For this review, take the finished solid that the model builds, in its own axes (mm). Face numbers are marked on the shaded views. A direction names the side the tool comes from. Round coordinates to 2 decimals unless told otherwise and drop trailing zeros. Write each loop counter-clockwise with the first axis right and the second up, starting at its lowest first coordinate (ties: lowest second). Pieces come first, ordered by that corner, then holes. Notation, with made-up numbers: M 55.25,5 L 67.25,5 A11 cw 67.25,26 Z; hole C -30.75,14 d2. An arc over 180 degrees is marked long. Answer in a Markdown table with one row per item.
```python
from build123d import *

# Parameters (mm, degrees)
SKETCH1_W           = 40
SKETCH1_H           = 40
BOSS_EXTRUDE1_DEPTH = 1.5
SKETCH2_R           = 7
BOSS_EXTRUDE2_DEPTH = 6


with BuildPart() as part:
    # Sketch1 → Boss-Extrude1 (new body)
    with BuildSketch(Plane(origin=(0, 0, 0), x_dir=(1, 0, 0), z_dir=(0, 1, 0))):
        with Locations((0, 20)):
            Rectangle(SKETCH1_W, SKETCH1_H)
    extrude(amount=BOSS_EXTRUDE1_DEPTH)

    # Sketch2 → Boss-Extrude2 (add)
    with BuildSketch(Plane(origin=(0, 1.5, 0), x_dir=(1, 0, 0), z_dir=(0, 1, 0))):
        with Locations(Location((0, 20, 0), (0, 0, 270))):
            Circle(SKETCH2_R)
        with BuildLine():
            ThreePointArc((-6.787334683, 32.2446759), (0, 34), (6.787334683, 32.2446759))
            ThreePointArc((6.787334683, 32.2446759), (8.731496224, 32.882040662), (8.241763544, 34.868535021))
            ThreePointArc((8.241763544, 34.868535021), (0, 37), (-8.241763544, 34.868535021))
            ThreePointArc((-8.241763544, 34.868535021), (-8.731496224, 32.882040662), (-6.787334683, 32.2446759))
        make_face()
        with BuildLine():
            ThreePointArc((-8.241763544, 5.131464979), (0, 3), (8.241763544, 5.131464979))
            ThreePointArc((8.241763544, 5.131464979), (8.731496224, 7.117959338), (6.787334683, 7.7553241))
            ThreePointArc((6.787334683, 7.7553241), (0, 6), (-6.787334683, 7.7553241))
            ThreePointArc((-6.787334683, 7.7553241), (-8.731496224, 7.117959338), (-8.241763544, 5.131464979))
        make_face()
        with BuildLine():
            ThreePointArc((12.2446759, 26.787334683), (14, 20), (12.2446759, 13.212665317))
            ThreePointArc((12.2446759, 13.212665317), (12.82939103, 11.173521325), (14.868535021, 11.758236456))
            ThreePointArc((14.868535021, 11.758236456), (17, 20), (14.868535021, 28.241763544))
            ThreePointArc((14.868535021, 28.241763544), (12.82939103, 28.826478675), (12.2446759, 26.787334683))
        make_face()
        with BuildLine():
            ThreePointArc((-12.2446759, 26.787334683), (-14, 20), (-12.2446759, 13.212665317))
            ThreePointArc((-12.2446759, 13.212665317), (-12.82939103, 11.173521325), (-14.868535021, 11.758236456))
            ThreePointArc((-14.868535021, 11.758236456), (-17, 20), (-14.868535021, 28.241763544))
            ThreePointArc((-14.868535021, 28.241763544), (-12.82939103, 28.826478675), (-12.2446759, 26.787334683))
        make_face()
    extrude(amount=BOSS_EXTRUDE2_DEPTH)


solid = part.part
```
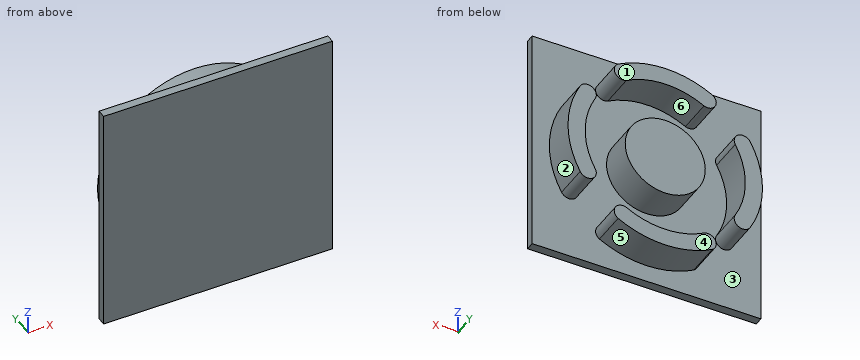
Q1. Take a section at C-C (z = -6.5). State the section outline as (x, y) points.
Found:
| item | result |
|---|---|
| outline | M -20,0 L 20,0 L 20,1.5 L 8.92,1.5 L 8.92,7.5 L 3.71,7.5 L 3.71,1.5 L -3.71,1.5 L -3.71,7.5 L -8.92,7.5 L -8.92,1.5 L -20,1.5 Z |
Q2. Take a section at B-B (x = 0). State the section outline as (y, z) points, then the cut area to 3 significant figures.
Found:
| item | result |
|---|---|
| outline | M 0,-40 L 1.5,-40 L 1.5,-37 L 7.5,-37 L 7.5,-34 L 1.5,-34 L 1.5,-27 L 7.5,-27 L 7.5,-13 L 1.5,-13 L 1.5,-6 L 7.5,-6 L 7.5,-3 L 1.5,-3 L 1.5,0 L 0,0 Z |
| area | 180 mm² |
Q3. Take a section at A-A (y = 5.25). State the section outline as (x, z) points.
Found:
| item | result |
|---|---|
| outline | M -14.87,-28.24 A1.5 ccw -12.24,-26.79 A14 cw -12.24,-13.21 A1.5 ccw -14.87,-11.76 A17 ccw Z; M -8.24,-34.87 A17 ccw 8.24,-34.87 A1.5 ccw 6.79,-32.24 A14 cw -6.79,-32.24 A1.5 ccw Z; M -8.24,-5.13 A1.5 ccw -6.79,-7.76 A14 cw 6.79,-7.76 A1.5 ccw 8.24,-5.13 A17 ccw Z; C 0,-20 d14; M 12.24,-26.79 A1.5 ccw 14.87,-28.24 A17 ccw 14.87,-11.76 A1.5 ccw 12.24,-13.21 A14 cw Z |
Q4. Take a section at D-D (z = -20). State the section outline as (x, y) points, then the cut area to 3 significant figures.
Found:
| item | result |
|---|---|
| outline | M -20,0 L 20,0 L 20,1.5 L 17,1.5 L 17,7.5 L 14,7.5 L 14,1.5 L 7,1.5 L 7,7.5 L -7,7.5 L -7,1.5 L -14,1.5 L -14,7.5 L -17,7.5 L -17,1.5 L -20,1.5 Z |
| area | 180 mm² |
Q5. For probe 1 along X at (y, z) = (3, -20); probe 2 along X at (y, z) = (4.25, -18); probe 3 along Z at (x, y) = (-0.5, 5.5), list the stretches that pass through material, from the lowest coordinate up.
Found:
| item | result |
|---|---|
| probe 1 | -17 to -14, -7 to 7, 14 to 17 |
| probe 2 | -16.88 to -13.86, -6.71 to 6.71, 13.86 to 16.88 |
| probe 3 | -36.99 to -33.99, -26.98 to -13.02, -6.01 to -3.01 |
Q6. Insertion check: P1, Ø2, axis at y = 5, z = -19.5, coming from the -X side. The pin has a flat end and moves straight along its axis. Give the tip position at first contact, or say it passes through.
Found:
| item | result |
|---|---|
| P1 | x = -17 |
Q7. Machinability: for the marked faces 4, 5 and 6, which of the approach directions +Z, -Z, +X, -X, +Y, -Y give a long, thin tool a straight path to every point of the face, cutting with its end or side? Answer none if there is none.
Found:
| item | result |
|---|---|
| face 4 | +Z, -Z, +X, -X, +Y |
| face 5 | -Z, +Y |
| face 6 | +Y |
Q8. Mouldability with a two-part tool opening along Z and no side actions: class the marked faces 1, 2 and 3 as +Z half, -Z half, draft (parallel to the pull), parting line (faces both ways), or undercut.
Found:
| item | result |
|---|---|
| face 1 | draft |
| face 2 | parting line |
| face 3 | undercut |
